```python
from build123d import *

# Parameters (mm, degrees)
SKETCH1_R              = 1.25
BOSS_EXTRUDE4_DEPTH    = 4
FILLET1_R              = 3.5
CUT_EXTRUDE1_START     = -31.73871501
CUT_EXTRUDE1_OUTLINE_R = 1.25
CUT_EXTRUDE1_DEPTH     = 3
CIRPATTERN1_COUNT      = 3


# Read off the part's stored shape, not the designer's step: Cut-Extrude1
with BuildPart() as part:
    # Sketch1 (on Front Plane) → Boss-Extrude4 (new body)
    with BuildSketch(Plane.XY):
        Polygon((0, 31.73871501), (-18.324355655, 31.73871501), (-27.486533482, 15.869357505), (-36.64871131, 0), (-27.486533482, -15.869357505), (-18.324355655, -31.73871501), (0, -31.73871501), (18.324355655, -31.73871501), (27.486533482, -15.869357505), (36.64871131, 0), (27.486533482, 15.869357505), (18.324355655, 31.73871501), align=None)
        Circle(SKETCH1_R, mode=Mode.SUBTRACT)
        Polygon((-2, 3.464101615), (-2, 27.73871501), (-16.014954578, 27.73871501), (-23.022431867, 15.601408313), align=None, mode=Mode.SUBTRACT)
        Polygon((-4, 0), (-25.022431867, -12.137306697), (-32.029909156, 0), (-25.022431867, 12.137306697), align=None, mode=Mode.SUBTRACT)
        Polygon((2, 27.73871501), (16.014954578, 27.73871501), (23.022431867, 15.601408313), (2, 3.464101615), align=None, mode=Mode.SUBTRACT)
        Polygon((25.022431867, 12.137306697), (32.029909156, 0), (25.022431867, -12.137306697), (4, 0), align=None, mode=Mode.SUBTRACT)
        Polygon((23.022431867, -15.601408313), (16.014954578, -27.73871501), (2, -27.73871501), (2, -3.464101615), align=None, mode=Mode.SUBTRACT)
        Polygon((-2, -3.464101615), (-2, -27.73871501), (-16.014954578, -27.73871501), (-23.022431867, -15.601408313), align=None, mode=Mode.SUBTRACT)
    extrude(amount=BOSS_EXTRUDE4_DEPTH)

    # Fillet1
    fillet1_edges = [part.edges().sort_by_distance(p)[0] for p in [
        (2, -27.73871501, 2),
        (16.014954578, -27.73871501, 2),
        (23.022431867, -15.601408313, 2),
        (2, -3.464101615, 2),
        (18.324355655, 31.73871501, 2),
        (36.64871131, 0, 2),
        (18.324355655, -31.73871501, 2),
        (-18.324355655, -31.73871501, 2),
        (-36.64871131, 0, 2),
        (-18.324355655, 31.73871501, 2),
        (23.022431867, 15.601408313, 2),
        (16.014954578, 27.73871501, 2),
        (2, 27.73871501, 2),
        (2, 3.464101615, 2),
        (-16.014954578, 27.73871501, 2),
        (-23.022431867, 15.601408313, 2),
        (-2, 3.464101615, 2),
        (-2, 27.73871501, 2),
        (-25.022431867, 12.137306697, 2),
        (-32.029909156, 0, 2),
        (-25.022431867, -12.137306697, 2),
        (-4, 0, 2),
        (25.022431867, -12.137306697, 2),
        (32.029909156, 0, 2),
        (25.022431867, 12.137306697, 2),
        (4, 0, 2),
        (-2, -3.464101615, 2),
        (-23.022431867, -15.601408313, 2),
        (-16.014954578, -27.73871501, 2),
        (-2, -27.73871501, 2),
    ]]
    fillet(fillet1_edges, radius=FILLET1_R)

    # Cut-Extrude1 outline → Cut-Extrude1 (cut)
    with BuildSketch(Plane(origin=(0, 0, 0), x_dir=(0.49999999999999195, -0.8660254037844434, 0), z_dir=(0.8660254037844433, 0.4999999999999921, 0)).offset(CUT_EXTRUDE1_START)):
        with Locations((15, -2)):
            Circle(CUT_EXTRUDE1_OUTLINE_R)
        with Locations((-15, -2)):
            Circle(CUT_EXTRUDE1_OUTLINE_R)
    cut_extrude1 = extrude(amount=CUT_EXTRUDE1_DEPTH, mode=Mode.SUBTRACT)

    # CirPattern1: Cut-Extrude1 ×3 about axis
    cirpattern1_axis = Axis((0, 0, 0), (0, 0, -1))
    for i in range(1, CIRPATTERN1_COUNT):
        add(cut_extrude1.rotate(cirpattern1_axis, i * 360 / CIRPATTERN1_COUNT), mode=Mode.SUBTRACT)


solid = part.part
```
Design review of the part built by this model. Coordinates are the model's own, in mm. A direction names the side the tool comes from. Round coordinates to 2 decimals unless told otherwise and drop trailing zeros. Write each loop counter-clockwise with the first axis right and the second up, starting at its lowest first coordinate (ties: lowest second). Pieces come first, ordered by that corner, then holes. Notation, with made-up numbers: (55, 57.5) -> (65, 57.5) arc R29 ccw to (65, 82.5) -> close; hole circle Ø1 at (-7.75, 17.5). An arc over 180 degrees is marked (long way). Write item = value, one per line. Start each with the question number.
1) Wall thickness on probe 1 along Y at (x, z) = (-5.5, 3.6); probe 2 along Z at (x, y) = (-15, 30.8); probe 3 along Y at (x, z) = (-9, 1.3): over which ranges is each line inside the solid? List them lowest first. Write a range as from..to.
2) Mouldability with a two-part tool opening along Y and no side actions: class faces 1 (the face through (-10, -27.739, 2)), 2 (the face through (13.81, 30.26, 1.62)), 3 (the face through (0, 31.739, 2)) as +Y half, -Y half, draft (parallel to the pull), parting line (faces both ways), or undercut.
3) Take a section at C-C, the plane x = 15. State the section outline as (y, z) points.
4) Take a section at D-D, the plane y = 20. State the section outline as (x, z) points.
5) Clearance check with flat-ended pins moving along their axes: pin 1 (1.2 mm diameter, centred on y = 16.5, z = 1.5, fed in from -X); pin 2 (1.5 mm diameter, centred on x = -15, z = 2, fed in from +Y); pin 3 (1.5 mm diameter, centred on y = 15, z = 2.5, fed in from +X). State where each tip first meets the part, or that it passes through.
6) Take a section at A-A, the plane x = 0. State the section outline as (y, z) points.
7) Tool access review of faces 4 (the face through (-17.4, -27.34, 1.98)), 5 (the face through (-3, 26.69, 2.03)), 6 (the face through (36.107, 0.026, 2.028)): name each direction out of +Z, -Z, +X, -X, +Y, -Y from which nothing blocks a thin tool from reaching the whole face with its end or side.
8) Take a section at B-B, the plane y = 13. State the section outline as (x, z) points, plus the area to 3 significant figures.
Results list:
q1.probe_1 = -31.74..-27.74, -6.03..6.03, 27.74..31.74
q1.probe_2 = 0..0.75, 3.25..4
q1.probe_3 = -31.74..-27.74, -7.51..-2.87, 2.87..7.51, 27.74..31.74
q2.face_1 = undercut
q2.face_2 = draft
q2.face_3 = +Y half
q3.outline = (-31.74, 0) -> (-27.59, 0) -> (-27.59, 4) -> (-31.74, 4) -> close; (-10.97, 0) -> (-6.35, 0) -> (-6.35, 4) -> (-10.97, 4) -> close; (6.35, 0) -> (10.97, 0) -> (10.97, 4) -> (6.35, 4) -> close; (27.59, 0) -> (31.74, 0) -> (31.74, 0.75) -> (28.74, 0.75) -> (28.74, 3.25) -> (31.74, 3.25) -> (31.74, 4) -> (27.59, 4) -> close
q4.outline = (-25.1, 0) -> (-20.48, 0) -> (-20.48, 4) -> (-25.1, 4) -> close; (-2, 0) -> (2, 0) -> (2, 4) -> (-2, 4) -> close; (20.48, 0) -> (25.1, 0) -> (25.1, 4) -> (20.48, 4) -> close
q5.pin_1 = -27.47
q5.pin_2 = 28.74
q5.pin_3 = 28.42
q6.outline = (-31.74, 0) -> (-1.25, 0) -> (-1.25, 4) -> (-31.74, 4) -> close; (1.25, 0) -> (31.74, 0) -> (31.74, 4) -> (1.25, 4) -> close
q7.face_4 = none
q7.face_5 = +Z, -Z
q7.face_6 = +Z, -Z, +X
q8.outline = (-29.14, 0) -> (-18.52, 0) -> (-18.52, 4) -> (-29.14, 4) -> close; (-2, 0) -> (2, 0) -> (2, 4) -> (-2, 4) -> close; (18.52, 0) -> (29.14, 0) -> (29.14, 4) -> (18.52, 4) -> close
q8.area = 101 mm²
